Check sheet for the drawn part. Datum: minimum x, y, z corner. Units: mm. Round coordinates to 2 decimals unless told otherwise and drop trailing zeros. Loops run counter-clockwise (first coordinate to the right, second up) from the corner with the lowest first, then second, coordinate; pieces in that order, holes last. Notation, with made-up numbers: (85, 29) -> (96, 29) arc R34 ccw to (96, 64) -> close; hole circle Ø5 at (-26.75, 88.5). An arc over 180 degrees is marked (long way). Write item = value, one per line. Start each with the question number.
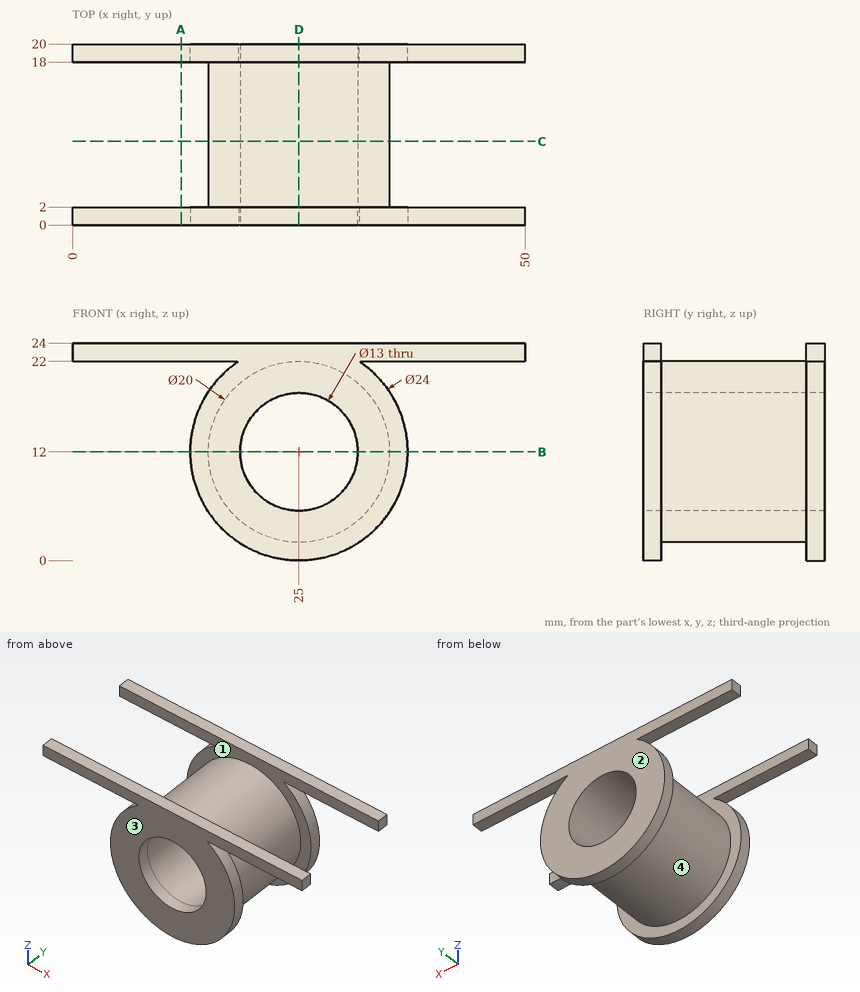
(1) Draft check along Y on the marked faces 1, 2, 3 and 4. Enter one of: +Y half, -Y half, draft (parallel to the pull), parting line (faces both ways), or undercut.
(2) Depth check by flat-ended pin: pin 1 Ø1 at (x, y) = (20, 7.5) entering from +Z; pin 2 Ø1 at (y, z) = (4.5, 13) entering from -X; pin 3 Ø10 at (y, z) = (2.5, 13.5) entering from -X; pin 4 Ø8 at (x, z) = (25, 12) entering from +Y. Enter the tip coordinate at first touch or a pass-through.
(3) Section check A-A on x = 12. Enter the section's corners in (y, z), then the cut area to 3 significant figures.
(4) Section check B-B on z = 12. Enter the section's corners in (x, y).
(5) Section check C-C on y = 9.25. Enter the section's corners in (x, z).
(6) Scan lines: line 1 (Z direction, x = 25, y = 1); line 2 (Y direction, x = 23, z = 22.25); line 3 (Z direction, x = 28, y = 12.25). Record each from-to range of solid material in increasing order. Write a range as [from, to].
(7) Section check D-D on x = 25. Enter the section's corners in (y, z).
Computed values:
q1.face_1 = undercut
q1.face_2 = +Y half
q1.face_3 = -Y half
q1.face_4 = undercut
q2.pin_1 = 20.93
q2.pin_2 = 15.01
q2.pin_3 = 13
q2.pin_4 = through
q3.outline = (0, 22) -> (2, 22) -> (2, 24) -> (0, 24) -> close; (18, 22) -> (20, 22) -> (20, 24) -> (18, 24) -> close
q3.area = 8.00 mm²
q4.outline = (13, 0) -> (18.5, 0) -> (18.5, 20) -> (13, 20) -> (13, 18) -> (15, 18) -> (15, 2) -> (13, 2) -> close; (31.5, 0) -> (37, 0) -> (37, 2) -> (35, 2) -> (35, 18) -> (37, 18) -> (37, 20) -> (31.5, 20) -> close
q5.outline = circle Ø20 at (25, 12); hole circle Ø13 at (25, 12)
q6.line_1 = [0, 5.5], [18.5, 24]
q6.line_2 = [0, 2], [18, 20]
q6.line_3 = [2.46, 6.23], [17.77, 21.54]
q7.outline = (0, 0) -> (2, 0) -> (2, 2) -> (18, 2) -> (18, 0) -> (20, 0) -> (20, 5.5) -> (0, 5.5) -> close; (0, 18.5) -> (20, 18.5) -> (20, 24) -> (18, 24) -> (18, 22) -> (2, 22) -> (2, 24) -> (0, 24) -> close
